Input: part model. Units: mm. Frame: model coordinates. A direction names the side the tool comes from. Coordinates: 2 decimals unless noted, no trailing zeros. Order: outer loops, then holes, each group sorted by start corner. A loop starts at its lowest first (then second) coordinate and runs counter-clockwise, first axis right, second up. Notation, with made-up numbers: (32, 30.5) -> (45, 30.5) arc R14 cw to (45, 39.5) -> close; hole circle Ø5 at (7, 3.25). An arc over 180 degrees is marked (long way). One line per item, written item: value. Start each with the question number.
from build123d import *

# Parameters (mm, degrees)
BOSS_EXTRUDE1_DEPTH     = 70
SKETCH3_R               = 4.1
CUT_EXTRUDE2_DEPTH      = 36.5
CUT_EXTRUDE2_DEPTH_BACK = 36.5
BOSS_EXTRUDE2_DEPTH     = 70
BOSS_EXTRUDE5_DEPTH     = 70
BOSS_EXTRUDE6_DEPTH     = 21
CHAMFER1_SIZE           = 20
CHAMFER4_SIZE           = 1


with BuildPart() as part:
    # Sketch1 → Boss-Extrude1 (new body)
    with BuildSketch(Plane(origin=(0, 0, 0), x_dir=(0, 0, -1), z_dir=(1, 0, 0))):
        Polygon((-30.5, 0), (-30.5, 20), (-30.5, 98), (30.5, 98), (30.5, 0), (35.5, 0), (35.5, 108), (-35.5, 108), (-35.5, 0), align=None)
    extrude(amount=-BOSS_EXTRUDE1_DEPTH)

    # Sketch3 → Cut-Extrude2 (cut, two sides)
    with BuildSketch(Plane.XY) as cut_extrude2_sk:
        with Locations((-60, 10)):
            Circle(SKETCH3_R)
        with Locations((-10, 10)):
            Circle(SKETCH3_R)
    extrude(amount=CUT_EXTRUDE2_DEPTH, mode=Mode.SUBTRACT)
    extrude(cut_extrude2_sk.sketch, amount=-CUT_EXTRUDE2_DEPTH_BACK, mode=Mode.SUBTRACT)

    # Sketch4 → Boss-Extrude2 (add)
    with BuildSketch(Plane(origin=(0, 0, 0), x_dir=(0, 0, -1), z_dir=(1, 0, 0))):
        Polygon((-30.5, 98), (-10.5, 98), (-16.5, 79.151), (-30.5, 79.151), align=None)
    boss_extrude2 = extrude(amount=-BOSS_EXTRUDE2_DEPTH)

    # Mirror2: Boss-Extrude2 across plane
    add(boss_extrude2.mirror(Plane.XY))

    # Sketch5 → Boss-Extrude5 (add)
    with BuildSketch(Plane.ZY.offset(70)):
        with BuildLine():
            Line((-30.5, 62.151), (-30.5, 79.151))
            Line((-30.5, 79.151), (-16.5, 79.151))
            ThreePointArc((-16.5, 79.151), (-14.785973083, 71.828090742), (-10, 66.026595252))
            Line((-10, 66.026595252), (-10, 62.151))
            Line((-10, 62.151), (-10, 58.045669043))
            ThreePointArc((-10, 58.045669043), (-19.497965112, 41.023297158), (-9.512195122, 24.282422523))
            Line((-9.512195122, 24.282422523), (-9.512195122, 20.305))
            Line((-9.512195122, 20.305), (-30.5, 20.305))
            Line((-30.5, 20.305), (-30.5, 41.305))
            Line((-30.5, 41.305), (-30.5, 62.151))
        make_face()
    boss_extrude5 = extrude(amount=-BOSS_EXTRUDE5_DEPTH)

    # Mirror3: Boss-Extrude5 across plane
    add(boss_extrude5.mirror(Plane.XY))

    # Sketch6 → Boss-Extrude6 (add)
    with BuildSketch(Plane(origin=(0, 0, 0), x_dir=(0, 0, -1), z_dir=(1, 0, 0))):
        with BuildLine():
            Line((-9.512195122, 20.305), (9.512195122, 20.305))
            Line((9.512195122, 20.305), (9.512195122, 24.282422523))
            ThreePointArc((9.512195122, 24.282422523), (19.497965112, 41.023297158), (10, 58.045669043))
            Line((10, 58.045669043), (-10, 58.045669043))
            ThreePointArc((-10, 58.045669043), (-19.497965112, 41.023297158), (-9.512195122, 24.282422523))
            Line((-9.512195122, 24.282422523), (-9.512195122, 20.305))
        make_face()
    extrude(amount=-BOSS_EXTRUDE6_DEPTH)

    # Mirror1: Boss-Extrude2 across plane
    add(boss_extrude2.mirror(Plane.XY))

    # Chamfer1
    chamfer1_edges = [part.edges().sort_by_distance(p)[0] for p in [
        (-35, 108, 35.5),
        (-35, 108, -35.5),
    ]]
    chamfer(chamfer1_edges, length=CHAMFER1_SIZE)

    # Chamfer4
    chamfer4_edges = [part.edges().sort_by_distance(p)[0] for p in [
        (-70, 41.023297158, 19.497965112),
        (-70, 62.036132147, 10),
        (-70, 71.828090742, 14.785973083),
        (-70, 98, 0),
        (-70, 88.5755, 13.5),
        (-70, 88.5755, -13.5),
        (-70, 41.023297158, -19.497965112),
        (-70, 62.036132147, -10),
        (-70, 71.828090742, -14.785973083),
    ]]
    chamfer(chamfer4_edges, length=CHAMFER4_SIZE)


solid = part.part
1) Section query B-B, the plane x = -60. State how many separate pieces and enclosed holes the cut face has, plus the area to 3 significant figures.
2) Pin query (flat end, axial travel): pin 1 Ø17 at (x, z) = (-26.5, 4) entering from -Y (3 decimals); pin 2 Ø3 at (x, z) = (-48.5, 4) entering from -Y; pin 3 Ø2 at (x, z) = (-32.5, -27) entering from +Y. Return the tip coordinate at first contact, or that it passes through.
3) Section query C-C, the plane z = 1. Return the cut outline in (x, y) (3 decimals).
4) Section query A-A, the plane y = 10. Return the cut outline in (x, z), plus the area to 3 significant figures.
5) Ray query, line 1 along X through (y, z) = (10, 31.7); line 2 along Z through (x, y) = (-28, 14.5); line 3 along Z through (x, y) = (-44, 41.5). Return the intervals inside material, ascending. Write a range as from..to.
6) Section query D-D, the plane y = 82. Return the cut outline in (x, z).
7) Mould query, pull axis X, two halves, no side actions, for faces 4 (the flat face through (0, 55, 0)), 5 (the cylindrical face through (-14.096, 10.18, 32.965)), 6 (the flat face through (-46, 22, -9.512)), 7 (the conical face through (-69.17, 71.92, -15.02)). Classes: +X half, -X half, draft (parallel to the pull), parting line (faces both ways), or undercut.
8) Access query for faces 1 (the flat face through (-35, 43, -35.5)), 2 (the flat face through (-34, 98, 0)), 3 (the cylindrical face through (-45.3, 41.3, 19.5)). Directions: +Z, -Z, +X, -X, +Y, -Y. A direction counts if a zero-diameter tool reaches every point of the face in a straight line with its end or side. Return the directions, or none.
Entries:
1. separate pieces: 3
1. enclosed holes: 0
1. area: 3,700 mm2
2. pin 1: stops at y = 20.305
2. pin 2: stops at y = 98
2. pin 3: stops at y = 97.5
3. outline: (-70, 99) -> (-69, 98) -> (0, 98) -> (0, 108) -> (-70, 108) -> close; (-21, 20.305) -> (0, 20.305) -> (0, 58.046) -> (-21, 58.046) -> close
4. outline: (-70, -35.5) -> (-64.1, -35.5) -> (-64.1, -30.5) -> (-70, -30.5) -> close; (-70, 30.5) -> (-64.1, 30.5) -> (-64.1, 35.5) -> (-70, 35.5) -> close; (-55.9, -35.5) -> (-14.1, -35.5) -> (-14.1, -30.5) -> (-55.9, -30.5) -> close; (-55.9, 30.5) -> (-14.1, 30.5) -> (-14.1, 35.5) -> (-55.9, 35.5) -> close; (-5.9, -35.5) -> (0, -35.5) -> (0, -30.5) -> (-5.9, -30.5) -> close; (-5.9, 30.5) -> (0, 30.5) -> (0, 35.5) -> (-5.9, 35.5) -> close
4. area: 536 mm2
5. line 1: x = -70..-64.1, -55.9..-14.1, -5.9..0
5. line 2: z = -35.5..-30.5, 30.5..35.5
5. line 3: z = -35.5..-19.5, 19.5..35.5
6. outline: (-70, -35.5) -> (0, -35.5) -> (0, -15.59) -> (-69, -15.59) -> (-70, -16.64) -> close; (-70, 16.64) -> (-69, 15.59) -> (0, 15.59) -> (0, 35.5) -> (-70, 35.5) -> close
7. face 4: +X half
7. face 5: undercut
7. face 6: draft
7. face 7: -X half
8. face 1: -Z, +X, -X, +Y, -Y
8. face 2: +X, -X
8. face 3: -X
